Drawing for the job (mm, zero at the part's lowest x, y, z). A direction names the side the tool comes from. Coordinates: 2 decimals unless noted, no trailing zeros. Order: outer loops, then holes, each group sorted by start corner. A loop starts at its lowest first (then second) coordinate and runs counter-clockwise, first axis right, second up.
1) Cut at B-B (z = 30). List the corners of the cut face in (x, y), and give its area (3 significant figures).
2) Cut at C-C (x = 36). List the corners of the cut face in (y, z), and give its area (3 significant figures).
3) Cut at A-A (y = 10). List the corners of the cut face in (x, z), and give its area (3 significant figures).
4) Wall check: L1, parallel to Z at x = 0.6, y = 25; L2, parallel to X at y = 43.5, z = 44. Give the ranges that are in metal, low to high.
5) Cut at D-D (y = 25). List the corners of the cut face in (x, z), and give its area (3 significant figures).
6) Pin check, flat tips, straight feed: pin 1 Ø5 at (x, y) = (14, 13) entering from -Z; pin 2 Ø2 at (y, z) = (16.5, 41) entering from +X; pin 3 Ø12 at (x, z) = (17.5, 11) entering from +Y. Stop position of each tip, or through.
7) Tool access for the marked faces 1 and 2: list every direction of +Z, -Z, +X, -X, +Y, -Y with a clear straight run to the whole face (end or side of a thin tool).
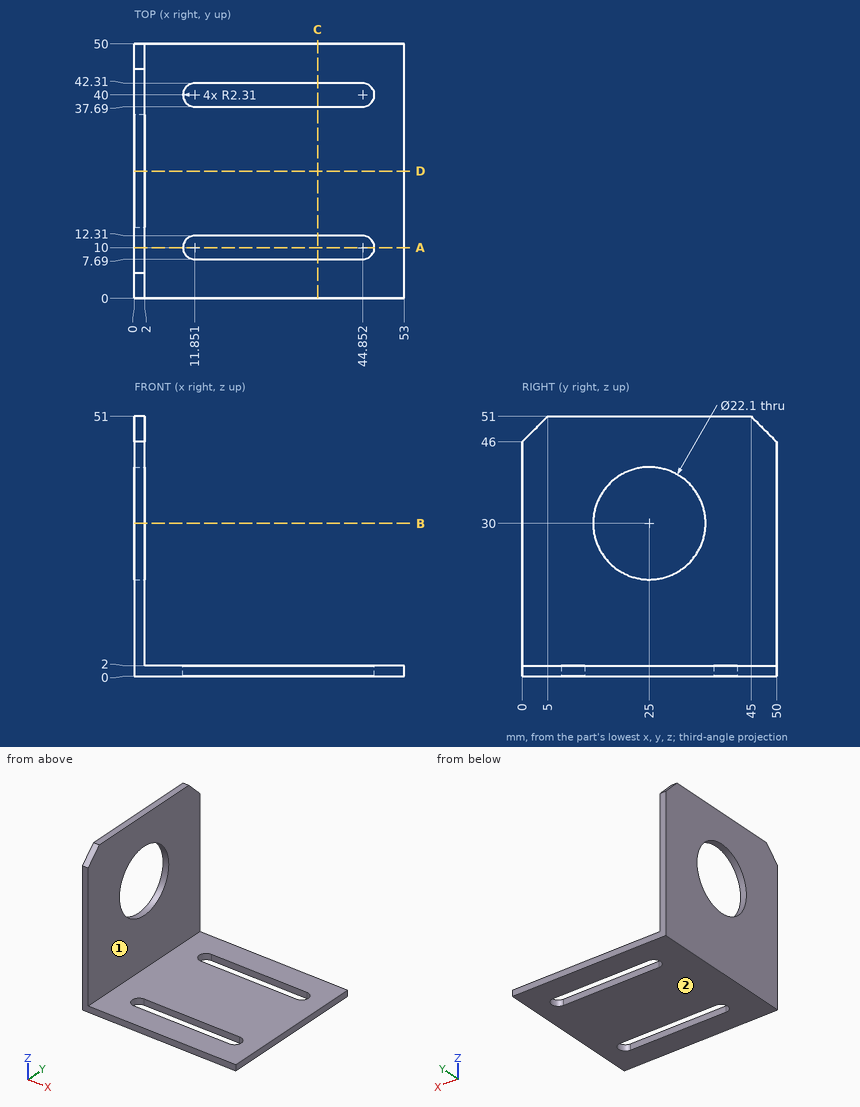
Geometry check:
1. outline: (0, 0) - (2, 0) - (2, 13.95) - (0, 13.95) - close; (0, 36.05) - (2, 36.05) - (2, 50) - (0, 50) - close
1. area: 55.8 mm2
2. outline: (0, 0) - (7.69, 0) - (7.69, 2) - (0, 2) - close; (12.31, 0) - (37.69, 0) - (37.69, 2) - (12.31, 2) - close; (42.31, 0) - (50, 0) - (50, 2) - (42.31, 2) - close
2. area: 81.5 mm2
3. outline: (0, 0) - (9.54, 0) - (9.54, 2) - (2, 2) - (2, 51) - (0, 51) - close; (47.16, 0) - (53, 0) - (53, 2) - (47.16, 2) - close
3. area: 129 mm2
4. L1: z = 0 to 18.95, 41.05 to 51
4. L2: x = 0 to 2
5. outline: (0, 0) - (53, 0) - (53, 2) - (2, 2) - (2, 18.95) - (0, 18.95) - close; (0, 41.05) - (2, 41.05) - (2, 51) - (0, 51) - close
5. area: 160 mm2
6. pin 1: stops at z = 0
6. pin 2: stops at x = 2
6. pin 3: passes through
7. face 1: +Z, +X, +Y, -Y
7. face 2: -Z, +X, -X, +Y, -Y
